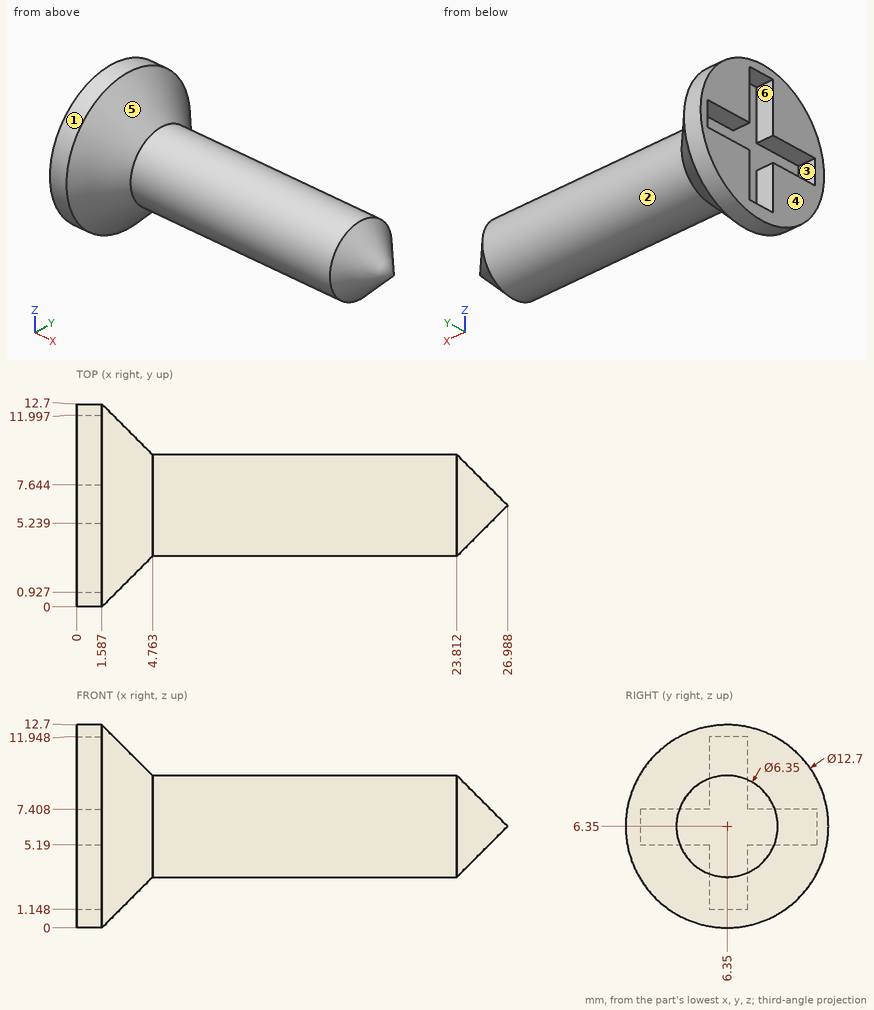
Could you check a few things on this drawing? It's one solid part, dimensions in mm from its lowest x, y, z. A direction names the side the tool comes from. Coordinates: 2 decimals unless noted, no trailing zeros.
1) We'd pull the mould along Y, two halves only. Please class the marked faces 4, 5 and 6: +Y half, -Y half, draft (parallel to the pull), parting line (faces both ways), or undercut.
2) Which directions (+Z, -Z, +X, -X, +Y, -Y) give clear straight access to the entire face, cutting with the end or side of a thin tool? Please do the marked faces 1, 2 and 3.
3) Will these pins go through, and if not, where does the flat tip stop? pin 1 (1.3 mm diameter, centred on x = 1, z = 3.5, fed in from -Y); pin 2 (1 mm diameter, centred on x = 17.5, y = 3, fed in from -Z); pin 3 (0.8 mm diameter, centred on x = 1, y = 2.5, fed in from +Z); pin 4 (1.5 mm diameter, centred on x = 21, y = 2, fed in from +Z).
4) I need wall thicknesses on line 1 (Y direction, x = 23.25, z = 6.5); line 2 (Z direction, x = 17, y = 7.25) (1 decimal). Which ranges of each line are inside material? Lowest first, please.
Response values:
1. face 4: draft
1. face 5: parting line
1. face 6: undercut
2. face 1: +X, -X
2. face 2: +X
2. face 3: -X
3. pin 1: stops at y = 0.39
3. pin 2: stops at z = 4.95
3. pin 3: stops at z = 11.68
3. pin 4: passes through
4. line 1: y = 3.18 to 9.52
4. line 2: z = 3.3 to 9.4
